```python
from build123d import *

# Parameters (mm, degrees)
SKETCH_2_R            = 25
SKETCH_2_R_2          = 1.5
EXTRUDE_1_DEPTH       = 2
CUT_EXTRUDE_2_REACH   = 44.732
SKETCH_5_W            = 45.82575695
SKETCH_5_H            = 15
HOLE_WIZARD_6_0_6_1_D = 6


with BuildPart() as part:
    # 草图1 → 旋转2 (revolve)
    with BuildSketch(Plane.XY, mode=Mode.PRIVATE) as revolve_2_sk:
        Polygon((4, 6), (0, 6), (0, 7), (-2, 7), (-2, 0), (22, 0), (22, 3), (22, 5.9), (20.6, 5.9), (20.6, 5.5), (19.6, 5.5), (19.6, 6), (15.6, 6), (15.6, 5.9), (4, 5.9), align=None)
    revolve(revolve_2_sk.sketch.rotate(Axis((-38.40520389, 0, 0), (1, 0, 0)), 90), axis=Axis((-38.40520389, 0, 0), (1, 0, 0)))

    # 草图2 → 凸台-拉伸1 (add)
    with BuildSketch(Plane.ZY.offset(2)):
        Circle(SKETCH_2_R)
        with Locations((-20, 7)):
            Circle(SKETCH_2_R_2, mode=Mode.SUBTRACT)
        with Locations(Location((20, 7, 0), (0, 0, 180))):
            Circle(SKETCH_2_R_2, mode=Mode.SUBTRACT)
        with Locations((20, -7)):
            Circle(SKETCH_2_R_2, mode=Mode.SUBTRACT)
        with Locations(Location((-20, -7, 0), (0, 0, 180))):
            Circle(SKETCH_2_R_2, mode=Mode.SUBTRACT)
    extrude(amount=EXTRUDE_1_DEPTH)

    # 草图5 → 切除-拉伸2 (cut, up to next)
    with BuildSketch(Plane(origin=(-2, 0, 0), x_dir=(0, 0, -1), z_dir=(1, 0, 0)), mode=Mode.PRIVATE) as cut_extrude_2_sk1:
        with Locations((0, 17.5)):
            Rectangle(SKETCH_5_W, SKETCH_5_H)
    cut_extrude_2_tool1 = extrude(cut_extrude_2_sk1.sketch, amount=-CUT_EXTRUDE_2_REACH, mode=Mode.PRIVATE) & part.part
    cut_extrude_2 = cut_extrude_2_tool1.solids().sort_by_distance((-2, 17.5, 0))[0]
    add(cut_extrude_2, mode=Mode.SUBTRACT)

    # 镜向1: 切除-拉伸2 across plane
    add(cut_extrude_2.mirror(Plane.ZX), mode=Mode.SUBTRACT)

    # Ø6.0 (6) 直径孔1 (through all)
    with Locations(Plane.ZY.offset(4)):
        with Locations((0, 0)):
            Hole(HOLE_WIZARD_6_0_6_1_D / 2)


solid = part.part
```
Could you check a few things on this model? Use its own coordinates, in mm. A direction names the side the tool comes from. Coordinates: 2 decimals unless noted, no trailing zeros. Loops run counter-clockwise (first coordinate to the right, second up) from the corner with the lowest first, then second, coordinate; pieces in that order, holes last.
1) Thinking about a two-plate mould opening in Z: for faces 1 (the face through (0, -2, -6)), 2 (the face through (21.29, -0.259, -5.894)), 3 (the face through (-2.99, 7.07, -21.5)), which applies, released by +Z, released by -Z, zero draft, split by the parting line, or undercut?
Reported:
face 1: zero draft
face 2: split by the parting line
face 3: undercut
2) Which directions (+Z, -Z, +X, -X, +Y, -Y) give clear straight access to the entire face, cutting with the end or side of a thin tool? Please do faces 4 (the face through (20.09, 5.37, -1.19)), 5 (the face through (-4, 5, 0)), 6 (the face through (1.972, -1.802, 5.723)).
Reported:
face 4: none
face 5: +Z, -Z, -X, +Y, -Y
face 6: +X
3) Please list where these lines run through material, in increasing order: line 1 along Y through (x, z) = (-2.8, 20); line 2 along X through (y, z) = (0.75, -9); line 3 along Z through (x, y) = (9.5, -1).
Reported:
line 1: y = -10 to -8.5, -5.5 to 5.5, 8.5 to 10
line 2: x = -4 to -2
line 3: z = -5.81 to -2.83, 2.83 to 5.81
4) Imagine slicing it at D-D (x = -1). List the corners of the cut face in (y, z) for me.
Reported:
outline: circle Ø14 at (0, 0); hole circle Ø6 at (0, 0)
5) Will these pins go through, and if not, where does the flat tip stop? pin 1 Ø4 at (y, z) = (-7, 20) entering from +X; pin 2 Ø4 at (x, y) = (6, 2) entering from -Z; pin 3 Ø12 at (x, z) = (4.5, 3) entering from -Y; pin 4 Ø2.5 at (y, z) = (7, -20) entering from -X (3 decimals).
Reported:
pin 1: stops at x = -2
pin 2: stops at z = -5.9
pin 3: stops at y = -7
pin 4: passes through
6) Imagine slicing it at A-A (z = -20). List the corners of the cut face in (x, y) for me, and give its area (3 significant figures).
Reported:
outline: (-4, -10) - (-2, -10) - (-2, -8.5) - (-4, -8.5) - close; (-4, -5.5) - (-2, -5.5) - (-2, 5.5) - (-4, 5.5) - close; (-4, 8.5) - (-2, 8.5) - (-2, 10) - (-4, 10) - close
area: 28.0 mm2
